Work out the finished part from the listing and answer in its coordinate system (mm). A direction names the side the tool comes from. Coordinates: 2 decimals unless noted, no trailing zeros. Write each loop counter-clockwise with the first axis right and the second up, starting at its lowest first coordinate (ties: lowest second). Pieces come first, ordered by that corner, then holes. Notation, with made-up numbers: (-6, 36.25) - (28, 36.25) arc R21 cw to (28, 56.25) - close; hole circle Ø4 at (61.25, 56). An arc over 180 degrees is marked (long way). Use a Markdown table: item, result. Add a question column.
(1) Given pin 1 Ø1.5 at (x, z) = (-5, 38) entering from +Y, flat-ended and moving along its own axis, determine where the tip first touches the part or whether it passes through.
(2) The part is cut by section C-C, the plane z = 66. Give the vertices of the cut face in (x, y), then the cut area to 3 significant figures.
(3) Find the intervals of material crossed by line 1 (X direction, y = 2, z = 58); line 2 (Z direction, x = 0, y = 60); line 3 (Y direction, x = -21, z = 17.5), in increasing order. Write a range as from..to.
(4) The part is cut by section A-A, the plane x = 0. Give the vertices of the cut face in (y, z), then the cut area to 3 significant figures.
(5) A tool of negligible diameter and unlimited length cuts with its end or side. For faces 1 (the face through (-1, -76.804, 37)), 2 (the face through (1.125, 55.375, 27.633)), 3 (the face through (-1, 42.954, 45)), from which of +Z, -Z, +X, -X, +Y, -Y can it reach the whole face along a straight path? Write none if from no direction.
(6) The part is cut by section B-B, the plane y = -52. Give the vertices of the cut face in (x, z).
(7) For a pull along X with two mould halves and no side action, classify faces 4 (the face through (-17, 45.454, 37)), 5 (the face through (-71.583, -17, 37)), 6 (the face through (-69.083, -16, 37)) as released by +X, released by -X, zero draft, split by the parting line, or undercut.
(8) The part is cut by section D-D, the plane x = -35.5. Give the vertices of the cut face in (y, z).
from build123d import *

# Parameters (mm, degrees)
F0_W     = 143.1653276086
F0_H     = 97.2580723464
F1_DEPTH = 25
F2_DEPTH = 25
F3_DEPTH = 25
F4_DEPTH = 25
F5_T     = -2.5
F6_R     = 10.6397034599
F7_DEPTH = 22
F8_T     = -2
F9_DEPTH = 25


with BuildPart() as f1:
    # F0 (on Top) → F1 (new body)
    with BuildSketch(Plane.XY):
        with Locations((3.7253e-06, -3.1754020602)):
            Rectangle(F0_W, F0_H)
    extrude(amount=F1_DEPTH)

    # F2 (add): faces of the model
    f2_faces = [f1.faces().sort_by_distance(p)[0] for p in [
        (3.7253e-06, -51.8044382334, 12.5),
        (3.7253e-06, 45.4536341131, 12.5),
    ]]
    extrude(f2_faces, amount=F2_DEPTH, dir=(0, -1, 0))

    # F3 (add): faces of the model
    f3_faces = [f1.faces().sort_by_distance(p)[0] for p in [
        (3.7253e-06, -15.6754020602, 25),
        (3.7253e-06, -15.6754020602, 0),
    ]]
    extrude(f3_faces, amount=F3_DEPTH, dir=(0, 0, 1))

    # F4 (add): faces of the model
    f4_faces = [f1.faces().sort_by_distance(p)[0] for p in [
        (3.7253e-06, -15.6754020602, 50),
        (3.7253e-06, -15.6754020602, 0),
    ]]
    extrude(f4_faces, amount=F4_DEPTH, dir=(0, 0, 1))

    # F5
    f5_openings = [f1.faces().sort_by_distance(p)[0] for p in [
        (4e-06, -15.675402, 0),
        (4e-06, -15.675402, 75),
    ]]
    offset(amount=F5_T, openings=f5_openings)

    # F6 (on face) → F7 (join)
    with BuildSketch(Plane(origin=(0, 45.4536341131, 0), x_dir=(-1, 0, 0), z_dir=(0, 1, 0))):
        with Locations((0, 36.1995995045)):
            Circle(F6_R)
    extrude(amount=F7_DEPTH)

    # F8
    f8_openings = [f1.faces().sort_by_distance(p)[0] for p in [
        (0, 67.453634, 36.1996),
    ]]
    offset(amount=F8_T, openings=f8_openings, kind=Kind.INTERSECTION)

    # F9 (cut): a face of the model
    f9_faces = [f1.faces().sort_by_distance(p)[0] for p in [
        (0, 44.9536341131, 36.1995995045),
    ]]
    extrude(f9_faces, amount=-F9_DEPTH, mode=Mode.SUBTRACT)


solid = f1.part
Model answer:
| question | item | result |
|---|---|---|
| 1 | pin 1 | y = -74.3 |
| 2 | outline | (-71.58, -76.8) - (71.58, -76.8) - (71.58, 45.45) - (-71.58, 45.45) - close; hole (-69.08, -74.3) - (69.08, -74.3) - (69.08, 42.95) - (-69.08, 42.95) - close |
| 2 | area | 1,300 mm^2 |
| 3 | line 1 | -71.58..-69.08, 69.08..71.58 |
| 3 | line 2 | 25.56..27.56, 44.84..46.84 |
| 3 | line 3 | -76.8..-74.3, 42.95..45.45 |
| 4 | outline | (-76.8, 0) - (-74.3, 0) - (-74.3, 75) - (-76.8, 75) - close; (42.95, 0) - (45.45, 0) - (45.45, 25.56) - (67.45, 25.56) - (67.45, 27.56) - (42.95, 27.56) - close; (42.95, 44.84) - (67.45, 44.84) - (67.45, 46.84) - (45.45, 46.84) - (45.45, 75) - (42.95, 75) - close |
| 4 | area | 420 mm^2 |
| 5 | face 1 | +Z, -Z, +X, -X, -Y |
| 5 | face 2 | +Y |
| 5 | face 3 | +Z, -Z |
| 6 | outline | (-71.58, 0) - (-69.08, 0) - (-69.08, 75) - (-71.58, 75) - close; (69.08, 0) - (71.58, 0) - (71.58, 75) - (69.08, 75) - close |
| 7 | face 4 | zero draft |
| 7 | face 5 | released by -X |
| 7 | face 6 | undercut |
| 8 | outline | (-76.8, 0) - (-74.3, 0) - (-74.3, 75) - (-76.8, 75) - close; (42.95, 0) - (45.45, 0) - (45.45, 75) - (42.95, 75) - close |
